Check sheet for the drawn part. Datum: minimum x, y, z corner. Units: mm. A direction names the side the tool comes from. Give positions to 0.01 mm unless a question says otherwise; leave off trailing zeros. Order: outer loops, then holes, each group sorted by start corner. A loop starts at its lowest first (then second) coordinate and runs counter-clockwise, first axis right, second up. Notation, with made-up numbers: (86.25, -2.75) - (145.25, -2.75) arc R12 ccw to (145.25, 5.25) - close; hole circle Ø5 at (63, -22.75). An arc over 180 degrees is marked (long way). Answer as a JSON object with one key per item and string values. Group by question number.
(1) Access from +Z, -Z, +X, -X, +Y, -Y to the whole of each face (thin tool, end or side, straight path). Record for the marked faces 4 and 5.
(2) Thickness scan on line 1 (Y direction, x = 84, z = 4.75); line 2 (Z direction, x = 29, y = 11.5); line 3 (Y direction, x = 45, z = 19). Record the ranges inside material, lowest first.
(3) Mould release check, pull along Y, two halves, no side actions. Record for the marked faces 1, 2 and 3: +Y half, -Y half, draft (parallel to the pull), parting line (faces both ways), or undercut.
(4) Section check B-B (z = 27). Record the boundary of the cut face in (x, y).
(5) Section check A-A (y = 4.5). Record the boundary of the cut face in (x, z), then the cut area to 3 significant figures.
(6) Section check D-D (x = 47). Record the boundary of the cut face in (y, z) (1 decimal), then the cut area to 3 significant figures.
(7) Depth check by flat-ended pin: pin 1 Ø8 at (x, y) = (12, 12) entering from +Z (1 decimal); pin 2 Ø5 at (x, z) = (53, 25.5) entering from -Y; pin 3 Ø2 at (x, z) = (84, 12) entering from -Y; pin 4 Ø13 at (x, y) = (62, 10.5) entering from +Z. Enter the tip coordinate at first touch or a pass-through.
(8) Section check C-C (y = 27). Record the boundary of the cut face in (x, z) (1 decimal), then the cut area to 3 significant figures.
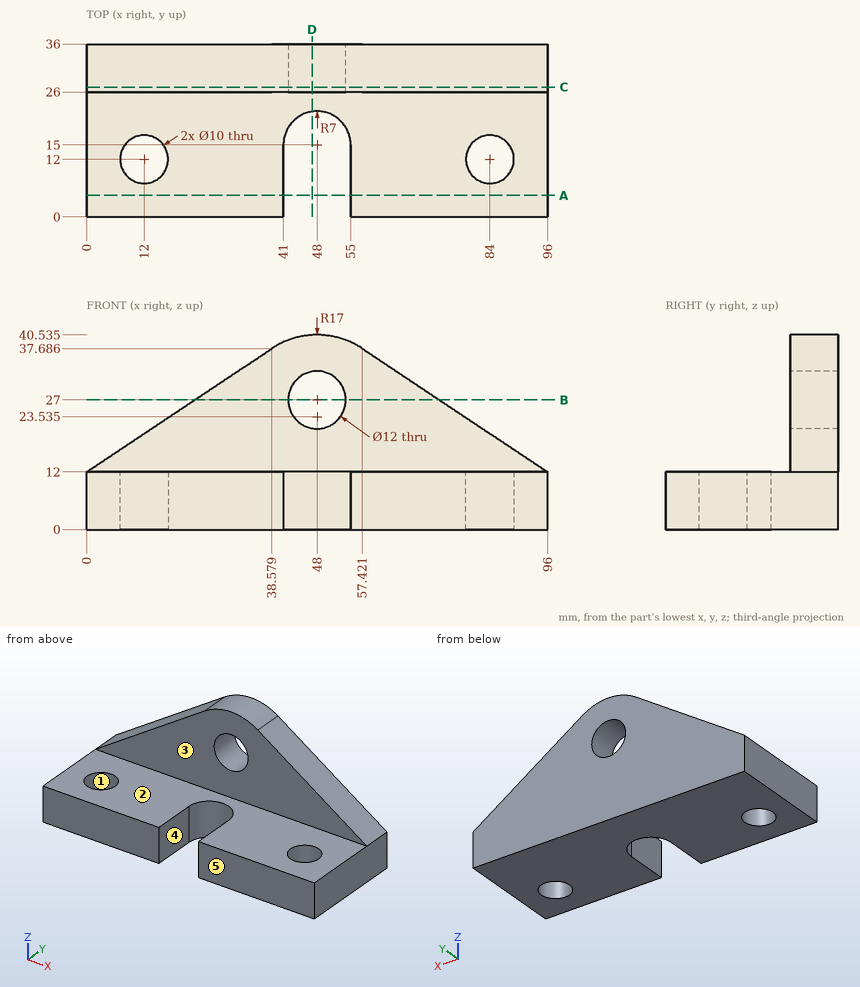
Solutions:
{
 "1": {"face 4": "+Z, -Z, -Y", "face 5": "+Z, -Z, +X, -X, -Y"},
 "2": {"line 1": "y = 0 to 7, 17 to 36", "line 2": "z = 0 to 12", "line 3": "y = 26 to 36"},
 "3": {"face 1": "undercut", "face 2": "draft", "face 3": "-Y half"},
 "4": {"outline": "(22.53, 26) - (42, 26) - (42, 36) - (22.53, 36) - close; (54, 26) - (73.47, 26) - (73.47, 36) - (54, 36) - close"},
 "5": {"outline": "(0, 0) - (41, 0) - (41, 12) - (0, 12) - close; (55, 0) - (96, 0) - (96, 12) - (55, 12) - close", "area": "984 mm2"},
 "6": {"outline": "(21.9, 0) - (36, 0) - (36, 21.1) - (26, 21.1) - (26, 12) - (21.9, 12) - close; (26, 32.9) - (36, 32.9) - (36, 40.5) - (26, 40.5) - close", "area": "336 mm2"},
 "7": {"pin 1": "passes through", "pin 2": "stops at y = 26", "pin 3": "stops at y = 0", "pin 4": "stops at z = 12"},
 "8": {"outline": "(0, 0) - (96, 0) - (96, 12) - (57.4, 37.7) arc R17 ccw to (38.6, 37.7) - (0, 12) - close; hole circle Ø12 at (48, 27)", "area": "2,550 mm2"}
}
